Source: CAD feature listing. Evaluate the final solid. Frame: model axes, mm. A direction names the side the tool comes from. Round coordinates to 2 decimals unless told otherwise and drop trailing zeros. Loops run counter-clockwise (first coordinate to the right, second up) from the corner with the lowest first, then second, coordinate; pieces in that order, holes last. Notation, with made-up numbers: (45, 33.25) - (79, 33.25) arc R14 cw to (79, 53.25) - close; hole circle Ø5 at (73, 13). An arc over 180 degrees is marked (long way). One line per question, with ' | ' between items. Start each with the question number.
1. Cut plane C-C (z = -51). Return loops of the section in (x, y).
2. Cut plane B-B (y = -56). Return loops of the section in (x, z), then the cut area to 3 significant figures.
3. Pin query (flat end, axial travel): pin 1 (4 mm diameter, centred on x = 10, y = -50.5, fed in from -Z); pin 2 (4 mm diameter, centred on x = -3.5, y = -64, fed in from -Z); pin 3 (1.5 mm diameter, centred on x = -13.5, z = -81, fed in from +Y). Return the tip coordinate at first contact, or that it passes through.
4. Cut plane A-A (x = 0). Return loops of the section in (y, z), then the cut area to 3 significant figures.
5. Access query for faces 1 (the cylindrical face through (15.978, -42.908, -79.691)), 2 (the flat face through (0, 0, 0)). Directions: +Z, -Z, +X, -X, +Y, -Y. A direction counts if a zero-diameter tool reaches every point of the face in a straight line with its end or side. Return the directions, or none.
6. Ray query, line 1 (X direction, y = -35.5, z = -96.5); line 2 (Y direction, x = -6.5, z = -34); line 3 (Z direction, x = -21, y = -29.5). Return the intervals inside material, ascending.
```python
from build123d import *

# Parameters (mm, degrees)
F0_R     = 27.469765
F1_DEPTH = 76.2
F2_R     = 17.296695
F3_DEPTH = 144.78
F4_R     = 5.08
F5_R     = 5.08
F6_R     = 5.08


with BuildPart() as f1:
    # F0 (on Front) → F1 (new body)
    with BuildSketch(Plane.XZ):
        Circle(F0_R)
    extrude(amount=F1_DEPTH)

    # F2 (on Top) → F3 (join)
    with BuildSketch(Plane.XY):
        with Locations((0, -36.283679)):
            Circle(F2_R)
    extrude(amount=-F3_DEPTH)

    # F4
    f4_edges = [f1.edges().sort_by_distance(p)[0] for p in [
        (-17.296695, -36.283679, -144.78),
    ]]
    fillet(f4_edges, radius=F4_R)

    # F5
    f5_edges = [f1.edges().sort_by_distance(p)[0] for p in [
        (-27.469765, 0, 0),
    ]]
    fillet(f5_edges, radius=F5_R)

    # F6
    f6_edges = [f1.edges().sort_by_distance(p)[0] for p in [
        (-27.469765, -76.2, 0),
    ]]
    fillet(f6_edges, radius=F6_R)


solid = f1.part
```
Answers follow:
1) outline: circle Ø34.59 at (0, -36.28)
2) outline: circle Ø54.94 at (0, 0) | area: 2,370 mm2
3) pin 1: stops at z = -143.67 | pin 2: stops at z = -27.43 | pin 3: stops at y = -24.6
4) outline: (-76.2, -22.39) arc R5.08 ccw to (-71.12, -27.47) - (-53.58, -27.47) - (-53.58, -139.7) arc R5.08 ccw to (-48.5, -144.78) - (-24.07, -144.78) arc R5.08 ccw to (-18.99, -139.7) - (-18.99, -27.47) - (-5.08, -27.47) arc R5.08 ccw to (0, -22.39) - (0, 22.39) arc R5.08 ccw to (-5.08, 27.47) - (-71.12, 27.47) arc R5.08 ccw to (-76.2, 22.39) - close | area: 8,210 mm2
5) face 1: -Z | face 2: +Z, -Z, +X, -X, +Y
6) line 1: x = -17.28 to 17.28 | line 2: y = -52.31 to -20.25 | line 3: z = -17.71 to 17.71
